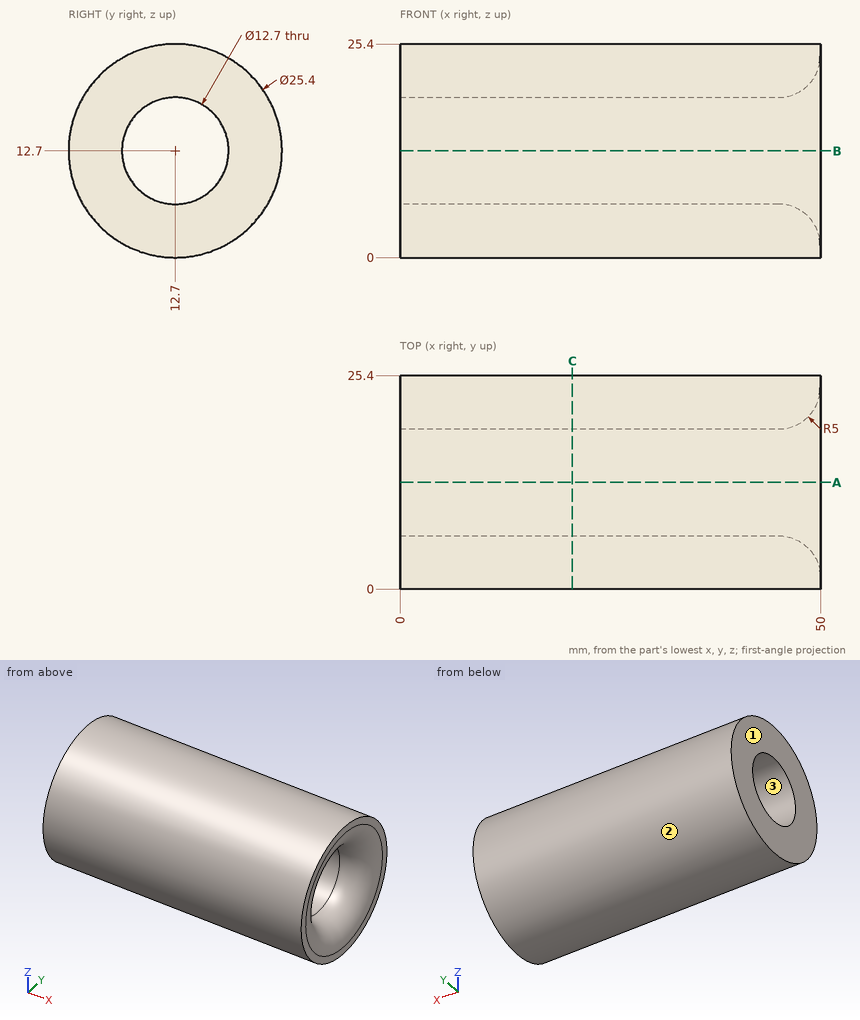
The drawing under review shows one solid part. Ordinate dimensions are in mm from its lowest x, y, z. Give positions to 0.01 mm unless a question says otherwise; leave off trailing zeros. Loops run counter-clockwise (first coordinate to the right, second up) from the corner with the lowest first, then second, coordinate; pieces in that order, holes last. Notation, with made-up numbers: M 72,82.5 L 76,82.5 A24 ccw 76,108.5 Z; hole C -4.5,8 d4. An arc over 180 degrees is marked long. Return JSON: item names as keys, results as strings. Group by question number.
Item 1: For probe 1 along Y at (x, z) = (23.5, 12.7); probe 2 along Z at (x, y) = (22, 14.5); probe 3 along X at (y, z) = (22, 6.5), list the stretches that pass through material, from the lowest coordinate up.
Item 2: Insertion check: pin 1 Ø12 at (y, z) = (17.5, 11.5) entering from +X; pin 2 Ø5 at (x, y) = (12.5, 7.5) entering from +Z; pin 3 Ø6 at (y, z) = (15.5, 18) entering from +X; pin 4 Ø6 at (x, y) = (37, 12) entering from +Z. Each pin has a flat end and moves straight along its axis. Give the tip position at first contact, or say it passes through.
Item 3: We need section C-C (x = 20.5). Give the boundary of the cut face in (y, z).
Item 4: We need section A-A (y = 12.7). Give the boundary of the cut face in (x, z).
Item 5: Mouldability with a two-part tool opening along Y and no side actions: class the marked faces 1, 2 and 3 as released by +Y, released by -Y, zero draft, split by the parting line, or undercut.
Output:
{
 "1": {"probe 1": "y = 0 to 6.35, 19.05 to 25.4", "probe 2": "z = 0.13 to 6.61, 18.79 to 25.27", "probe 3": "x = 0 to 50"},
 "2": {"pin 1": "stops at x = 49.98", "pin 2": "stops at z = 25.11", "pin 3": "stops at x = 49.41", "pin 4": "stops at z = 25.4"},
 "3": {"outline": "C 12.7,12.7 d25.4; hole C 12.7,12.7 d12.7"},
 "4": {"outline": "M 0,0 L 50,0 L 50,1.35 A5 ccw 45,6.35 L 0,6.35 Z; M 0,19.05 L 45,19.05 A5 ccw 50,24.05 L 50,25.4 L 0,25.4 Z"},
 "5": {"face 1": "zero draft", "face 2": "split by the parting line", "face 3": "undercut"}
}
